from build123d import *

# Parameters (mm, degrees)
BOSS_EXTRUDE1_DEPTH = 3.175
SKETCH2_R           = 1.5
CUT_EXTRUDE1_DEPTH  = 3.175


with BuildPart() as part:
    # Sketch1 → Boss-Extrude1 (new body)
    with BuildSketch(Plane.XY):
        Polygon((101.6, 279.4), (0, 279.4), (0, 260.883636364), (-3.175, 260.883636364), (-3.175, 244.72), (0, 244.72), (0, 228.563636364), (-3.175, 228.563636364), (-3.175, 212.4), (0, 212.4), (0, 196.243636364), (-3.175, 196.243636364), (-3.175, 180.08), (0, 180.08), (0, 163.923636364), (-3.175, 163.923636364), (-3.175, 147.76), (0, 147.76), (0, 131.603636364), (-3.175, 131.603636364), (-3.175, 115.44), (0, 115.44), (0, 99.283636364), (-3.175, 99.283636364), (-3.175, 83.12), (0, 83.12), (0, 66.963636364), (-3.175, 66.963636364), (-3.175, 50.8), (0, 50.8), (0, 34.64), (0, 0), (101.6, 0), (101.6, 34.64), (101.6, 50.8), (104.775, 50.8), (104.775, 66.963636364), (101.6, 66.963636364), (101.6, 83.12), (104.775, 83.12), (104.775, 99.283636364), (101.6, 99.283636364), (101.6, 115.44), (104.775, 115.44), (104.775, 131.603636364), (101.6, 131.603636364), (101.6, 147.76), (104.775, 147.76), (104.775, 163.923636364), (101.6, 163.923636364), (101.6, 180.08), (104.775, 180.08), (104.775, 196.243636364), (101.6, 196.243636364), (101.6, 212.4), (104.775, 212.4), (104.775, 228.563636364), (101.6, 228.563636364), (101.6, 244.72), (104.775, 244.72), (104.775, 260.883636364), (101.6, 260.883636364), align=None)
    extrude(amount=BOSS_EXTRUDE1_DEPTH)

    # Sketch2 → Cut-Extrude1 (cut)
    with BuildSketch(Plane.XY.offset(3.175)):
        with Locations((15.875, 20)):
            Circle(SKETCH2_R)
        with Locations((15.875, 35.75)):
            Circle(SKETCH2_R)
        with Locations((15.875, 243.65)):
            Circle(SKETCH2_R)
        with Locations((15.875, 259.4)):
            Circle(SKETCH2_R)
        with Locations((85.725, 259.4)):
            Circle(SKETCH2_R)
        with Locations((85.725, 243.65)):
            Circle(SKETCH2_R)
        with Locations((85.725, 35.75)):
            Circle(SKETCH2_R)
        with Locations((85.725, 20)):
            Circle(SKETCH2_R)
    extrude(amount=-CUT_EXTRUDE1_DEPTH, mode=Mode.SUBTRACT)


solid = part.part
Input: part model. Units: mm. Frame: model coordinates. Round coordinates to 2 decimals unless told otherwise and drop trailing zeros. Order: outer loops, then holes, each group sorted by start corner. A loop starts at its lowest first (then second) coordinate and runs counter-clockwise, first axis right, second up. Notation, with made-up numbers: (-18, 9) - (31, 9) arc R31 ccw to (31, 34) - close; hole circle Ø10 at (-32, 59). An arc over 180 degrees is marked (long way). Use a Markdown table: item, result.
1. Material intervals for probe 1 along Y at (x, z) = (15.5, 1.8); probe 2 along X at (y, z) = (243.65, 0.85) (3 decimals); probe 3 along X at (y, z) = (20.5, 2.05), sorted ascending.
Evaluation:
| item | result |
|---|---|
| probe 1 | 0 to 18.55, 21.45 to 34.3, 37.2 to 242.2, 245.1 to 257.95, 260.85 to 279.4 |
| probe 2 | 0 to 14.375, 17.375 to 84.225, 87.225 to 101.6 |
| probe 3 | 0 to 14.46, 17.29 to 84.31, 87.14 to 101.6 |
2. First-contact query: pin 1 (5 mm diameter, centred on x = 15.875, y = 20, fed in from -Z); pin 2 (1 mm diameter, centred on x = 104, z = 2, fed in from -Y); pin 3 (1.6 mm diameter, centred on y = 34, z = 2, fed in from -X); pin 4 (1 mm diameter, centred on x = 102.5, z = 2.5, fed in from +Y). Flat tips, straight axial feed; report the tip coordinate or a pass-through.
Evaluation:
| item | result |
|---|---|
| pin 1 | z = 0 |
| pin 2 | y = 50.8 |
| pin 3 | x = 0 |
| pin 4 | y = 260.88 |
3. Section B-B on y = 168.5. Return the cut outline in (x, z) (3 decimals), then the cut area to 3 significant figures.
Evaluation:
| item | result |
|---|---|
| outline | (0, 0) - (101.6, 0) - (101.6, 3.175) - (0, 3.175) - close |
| area | 323 mm^2 |
4. Section A-A on z = 2.45. State how many separate pieces and enclosed holes the cut face has, then the cut area to 3 significant figures.
Evaluation:
| item | result |
|---|---|
| separate pieces | 1 |
| enclosed holes | 8 |
| area | 29,000 mm^2 |
